Verification items for the finished model (mm, model axes). Face numbers are marked on the shaded views. A direction names the side the tool comes from. Round coordinates to 2 decimals unless told otherwise and drop trailing zeros. Order: outer loops, then holes, each group sorted by start corner. A loop starts at its lowest first (then second) coordinate and runs counter-clockwise, first axis right, second up. Notation, with made-up numbers: (36.25, 33.25) -> (51.25, 33.25) arc R27 ccw to (51.25, 60.25) -> close; hole circle Ø6 at (58, -0.5). An arc over 180 degrees is marked (long way). Return JSON: item names as keys, results as strings. Group by question number.
Item 1: Sectioned sample at A-A on z = 0. Record the cut outline in (x, y).
Item 2: Scan lines: probe 1 along X at (y, z) = (12.25, 0); probe 2 along Y at (x, z) = (5.75, 31.5); probe 3 along Y at (x, z) = (0.5, -23.5). Record each from-to range of solid material in increasing order. Write a range as from..to.
Item 3: Sectioned sample at D-D on x = -1.25. Record the cut outline in (y, z).
Item 4: Access from +Z, -Z, +X, -X, +Y, -Y to the whole of each face (thin tool, end or side, straight path). Record for the marked faces 5, 6, 7, 8 and 9.
Item 5: Depth check by flat-ended pin: pin 1 Ø2 at (x, z) = (-5, 0) entering from +Y; pin 2 Ø12 at (x, z) = (5, -13.5) entering from +Y; pin 3 Ø12 at (x, y) = (-2, -22) entering from -Z; pin 4 Ø8 at (x, y) = (-8, 5.5) entering from +Z. Enter the tip coordinate at first touch or a pass-through.
Item 6: Draft check along Y on the marked faces 1, 2, 3 and 4. Enter one of: pulls with the +Y half, pulls with the -Y half, needs draft (parallel to the pull), parting line crosses it, or undercut.
Item 7: Sectioned sample at B-B on y = 0. Record the cut outline in (x, z), plus the area to 3 significant figures.
Item 8: Sectioned sample at C-C on z = -30.5. Record the cut outline in (x, y), plus the area to 3 significant figures.
```python
from build123d import *

# Parameters (mm, degrees)
BASPROSKE_W             = 10
BASPROSKE_H             = 40
TOOTHCUT_DEPTH          = 58.445626465
TEETHCUTS_COUNT         = 14
HUBNEAONESKE_R          = 15
HUBNEARONE_DEPTH        = 10.0000508
BORSKE_R                = 8.5
BORE_DEPTH              = 20.0000508
CUT_EXTRUDE1_DEPTH      = 57.907695162
CUT_EXTRUDE1_DEPTH_BACK = 57.907695162
SKETCH1_R               = 1.75


with BuildPart() as part:
    # BasProSke → Base-Revolve (revolve)
    with BuildSketch(Plane(origin=(0, 0, 0), x_dir=(1, 0, 0), z_dir=(0, 1, 0)), mode=Mode.PRIVATE) as base_revolve_sk:
        with Locations((5, 20)):
            Rectangle(BASPROSKE_W, BASPROSKE_H)
    revolve(base_revolve_sk.sketch.rotate(Axis((-10, 0, 0), (1, 0, 0)), 180), axis=Axis((-10, 0, 0), (1, 0, 0)))

    # TooCutSke → ToothCut (cut, through all)
    with BuildSketch(Plane(origin=(0, 0, 0), x_dir=(0, 0, -1), z_dir=(1, 0, 0))):
        with BuildLine():
            ThreePointArc((2.668955068, 28.624843752), (0, 28.749), (-2.668955068, 28.624843752))
            ThreePointArc((-2.668955068, 28.624843752), (-4.092749085, 34.510467305), (-7.86881342, 39.244291566))
            ThreePointArc((-7.86881342, 39.244291566), (0, 40.0254), (7.86881342, 39.244291566))
            ThreePointArc((7.86881342, 39.244291566), (4.092749085, 34.510467305), (2.668955068, 28.624843752))
        make_face()
    toothcut = extrude(amount=TOOTHCUT_DEPTH, mode=Mode.SUBTRACT)

    # TeethCuts: ToothCut ×14 about axis
    teethcuts_axis = Axis((0, 0, 0), (1, 0, 0))
    for i in range(1, TEETHCUTS_COUNT):
        add(toothcut.rotate(teethcuts_axis, i * 360 / TEETHCUTS_COUNT), mode=Mode.SUBTRACT)

    # HubNeaOneSke → HubNearOne (add)
    with BuildSketch(Plane.ZY):
        with Locations(Location((0, 0, 0), (0, 0, 180))):
            Circle(HUBNEAONESKE_R)
    extrude(amount=HUBNEARONE_DEPTH)

    # BorSke → Bore (cut, symmetric)
    with BuildSketch(Plane(origin=(0, 0, 0), x_dir=(0, 0, -1), z_dir=(1, 0, 0))):
        with Locations(Location((0, 0, 0), (0, 0, 180))):
            Circle(BORSKE_R)
    extrude(amount=BORE_DEPTH, both=True, mode=Mode.SUBTRACT)

    # Sketch1 → Cut-Extrude1 (cut, two sides: drawn at the far end of the back side and taken through both)
    with BuildSketch(Plane(origin=(0, 0, 0), x_dir=(1, 0, 0), z_dir=(0, 1, 0)).offset(-CUT_EXTRUDE1_DEPTH_BACK)):
        with Locations(Location((-5.0000508, 0, 0), (0, 0, 270))):
            Circle(SKETCH1_R)
    extrude(amount=CUT_EXTRUDE1_DEPTH + CUT_EXTRUDE1_DEPTH_BACK, mode=Mode.SUBTRACT)


solid = part.part
```
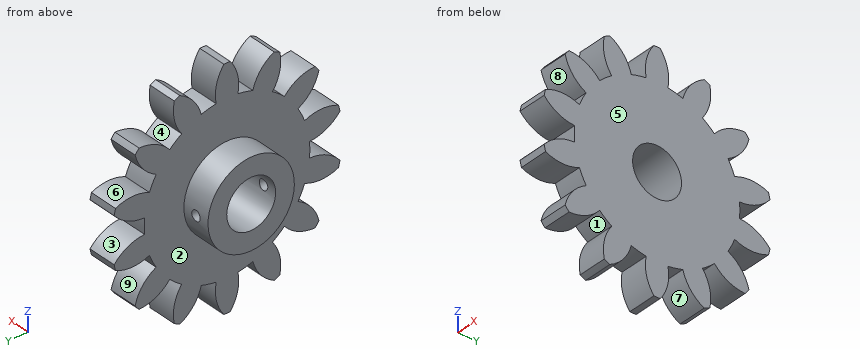
Recorded:
{
 "1": {"outline": "(-10, -15) -> (-6.75, -15) -> (-6.75, -8.5) -> (-10, -8.5) -> close; (-10, 8.5) -> (-6.75, 8.5) -> (-6.75, 15) -> (-10, 15) -> close; (-3.25, -15) -> (0, -15) -> (0, -28.75) -> (10, -28.75) -> (10, -8.5) -> (-3.25, -8.5) -> close; (-3.25, 8.5) -> (10, 8.5) -> (10, 28.75) -> (0, 28.75) -> (0, 15) -> (-3.25, 15) -> close"},
 "2": {"probe 1": "-10..-6.75, -3.25..10", "probe 2": "-18.61..-10.78, -4.06..4.06, 10.78..18.61", "probe 3": "-31.78..-23.06, -16.56..16.56, 23.06..31.78"},
 "3": {"outline": "circle Ø30 at (0, 0); hole circle Ø17 at (0, 0)"},
 "4": {"face 5": "+Z, -Z, +X, +Y, -Y", "face 6": "+X, -X", "face 7": "-Z, +X, -X", "face 8": "+X, -X, -Y", "face 9": "+X, -X, +Y"},
 "5": {"pin 1": "through", "pin 2": "y = 39.22", "pin 3": "z = -36.49", "pin 4": "z = 14.92"},
 "6": {"face 1": "undercut", "face 2": "needs draft", "face 3": "pulls with the +Y half", "face 4": "undercut"},
 "7": {"outline": "(-10, -15) -> (0, -15) -> (0, -40) -> (10, -40) -> (10, -8.5) -> (-10, -8.5) -> close; (-10, 8.5) -> (10, 8.5) -> (10, 40) -> (0, 40) -> (0, 15) -> (-10, 15) -> close", "area": "760 mm²"},
 "8": {"outline": "(0, -18.5) -> (10, -18.5) -> (10, -10.19) -> (0, -10.19) -> close; (0, -4.03) -> (10, -4.03) -> (10, 4.03) -> (0, 4.03) -> close; (0, 10.19) -> (10, 10.19) -> (10, 18.5) -> (0, 18.5) -> close", "area": "247 mm²"}
}
